For this review, take the finished solid that the model builds, in its own axes (mm). Face numbers are marked on the shaded views. A direction names the side the tool comes from. Give positions to 0.01 mm unless a question says otherwise; leave off trailing zeros. Write each loop counter-clockwise with the first axis right and the second up, starting at its lowest first coordinate (ties: lowest second). Pieces come first, ordered by that corner, then holes. Notation, with made-up numbers: M -11.75,51 L 44.25,51 A6 cw 44.25,60 Z; hole C -32,-21.75 d5. An arc over 180 degrees is marked long. Answer as a JSON object with one key per item and string values. Group by question number.
```python
from build123d import *

# Parameters (mm, degrees)
BOSS_EXTRU_1_DEPTH           = 100
ESQUISSE2_R                  = 1.75
ENL_V_MAT_EXTRU_1_DEPTH      = 101.238777427
ENL_V_MAT_EXTRU_2_DEPTH      = 101.238777427
ENL_V_MAT_EXTRU_2_DEPTH_BACK = 101.238777427
ESQUISSE3_W                  = 10.5
ESQUISSE3_H                  = 45
ENL_V_MAT_EXTRU_3_DEPTH      = 2.6


with BuildPart() as part:
    # Esquisse1 → Boss.-Extru.1 (new body)
    with BuildSketch(Plane.XY):
        Polygon((-2.25, 0), (2.25, 0), (5.25, 3), (5.25, 3.5), (2.45, 3.5), (2.45, 4.5), (-2.45, 4.5), (-2.45, 3.5), (-5.25, 3.5), (-5.25, 3), align=None)
    extrude(amount=BOSS_EXTRU_1_DEPTH)

    # Esquisse2 → Enlèv. mat.-Extru.1 (cut, through all)
    with BuildSketch(Plane(origin=(0, 4.5, 0), x_dir=(1, 0, 0), z_dir=(0, 1, 0))):
        with Locations(Location((0, -50, 0), (0, 0, 270))):
            Circle(ESQUISSE2_R)
    extrude(amount=-ENL_V_MAT_EXTRU_1_DEPTH, mode=Mode.SUBTRACT)

    # Esquisse3 → Enlèv. mat.-Extru.2 (cut, two sides: drawn at the far end of the back side and taken through both)
    with BuildSketch(Plane(origin=(0, 4.5, 0), x_dir=(1, 0, 0), z_dir=(0, 1, 0)).offset(-ENL_V_MAT_EXTRU_2_DEPTH_BACK)):
        with Locations((0, -77.5)):
            Rectangle(ESQUISSE3_W, ESQUISSE3_H)
        with Locations((0, -22.5)):
            Rectangle(ESQUISSE3_W, ESQUISSE3_H)
    extrude(amount=ENL_V_MAT_EXTRU_2_DEPTH + ENL_V_MAT_EXTRU_2_DEPTH_BACK, mode=Mode.SUBTRACT)

    # Esquisse4 → Enlèv. mat.-Extru.3 (cut)
    with BuildSketch(Plane.XZ):
        Polygon((2.85, 48.354551733), (2.85, 51.645448267), (0, 53.290896534), (-2.85, 51.645448267), (-2.85, 48.354551733), (0, 46.709103466), align=None)
    extrude(amount=-ENL_V_MAT_EXTRU_3_DEPTH, mode=Mode.SUBTRACT)


solid = part.part
```
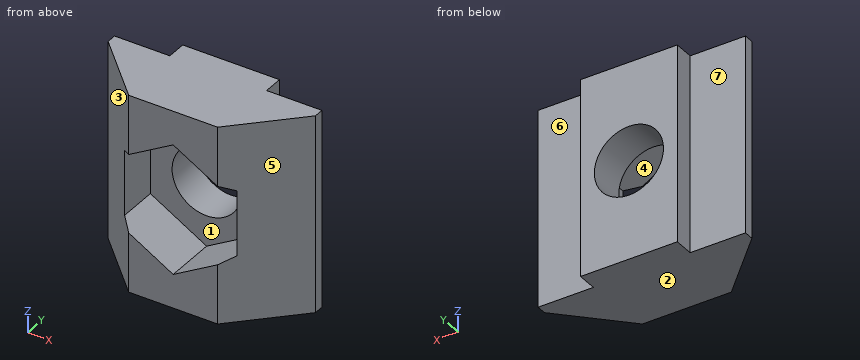
Item 1: Consider section D-D (y = 1.9). Give the boundary of the cut face in (x, z).
Item 2: Consider section B-B (z = 50). Give the boundary of the cut face in (x, y).
Item 3: Machinability: for the marked faces 4, 5, 6 and 7, which of the approach directions +Z, -Z, +X, -X, +Y, -Y give a long, thin tool a straight path to every point of the face, cutting with its end or side? Answer none if there is none.
Item 4: To check wall thickness, follow probe 1 along Y at (x, z) = (2.25, 48.75); probe 2 along Z at (x, y) = (1.5, 4); probe 3 along X at (y, z) = (3.9, 53.5). State the ranges of each line that lie inside material, in increasing order.
Item 5: Consider section A-A (y = 1.3). Give the boundary of the cut face in (x, z).
Item 6: Consider section C-C (x = -3.5). Give the boundary of the cut face in (y, z).
Item 7: Draft analysis for pull direction X (two halves, no side actions). For the marked faces 1, 2 and 3, state which applies: released by +X, released by -X, zero draft, split by the parting line, or undercut.
Item 8: Insertion check: P1, Ø3, axis at x = 1.5, z = 50.5, coming from the -Y side; P2, Ø0.8, axis at y = 4, z = 49, coming from the +X side; P3, Ø1, axis at y = 1.5, z = 50.5, coming from the -X side; P4, Ø2, axis at x = 0, z = 50, coming from the +Y side. Each pin has a flat end and moves straight along its axis. Give the tip position at first contact, or say it passes through.
Result set:
{
 "1": {"outline": "M -4.15,45 L 4.15,45 L 4.15,55 L -4.15,55 Z; hole M -2.85,48.35 L 0,46.71 L 2.85,48.35 L 2.85,51.65 L 0,53.29 L -2.85,51.65 Z"},
 "2": {"outline": "M -5.25,3 L -2.85,0.6 L -2.85,2.6 L -1.75,2.6 L -1.75,4.5 L -2.45,4.5 L -2.45,3.5 L -5.25,3.5 Z; M 1.75,2.6 L 2.85,2.6 L 2.85,0.6 L 5.25,3 L 5.25,3.5 L 2.45,3.5 L 2.45,4.5 L 1.75,4.5 Z"},
 "3": {"face 4": "-Y", "face 5": "+Z, -Z, +X, -Y", "face 6": "+Z, -Z, +X, +Y", "face 7": "+Z, -Z, -X, +Y"},
 "4": {"probe 1": "y = 2.6 to 4.5", "probe 2": "z = 45 to 49.1, 50.9 to 55", "probe 3": "x = -2.45 to 2.45"},
 "5": {"outline": "M -3.55,45 L 3.55,45 L 3.55,55 L -3.55,55 Z; hole M -2.85,48.35 L 0,46.71 L 2.85,48.35 L 2.85,51.65 L 0,53.29 L -2.85,51.65 Z"},
 "6": {"outline": "M 1.25,45 L 3.5,45 L 3.5,55 L 1.25,55 Z"},
 "7": {"face 1": "undercut", "face 2": "zero draft", "face 3": "released by -X"},
 "8": {"P1": "stops at y = 0.6", "P2": "stops at x = 2.45", "P3": "stops at x = -4.25", "P4": "passes through"}
}
